```python
from build123d import *

# Parameters (mm, degrees)
F0_W     = 50.8
F0_H     = 76.2
F1_DEPTH = 12.7
F3_DEPTH = 6.35
F4_R     = 3.175
F5_DEPTH = 12.701


with BuildPart() as f1:
    # F0 (on Front) → F1 (new body)
    with BuildSketch(Plane.XZ):
        with Locations((25.4, 38.1)):
            Rectangle(F0_W, F0_H)
    extrude(amount=F1_DEPTH)

    # F2 (on face) → F3 (cut)
    with BuildSketch(Plane.XZ.offset(12.7)):
        with BuildLine():
            Line((22.225, 63.5), (0, 63.5))
            Line((0, 63.5), (0, 57.15))
            Line((0, 57.15), (15.896593, 57.15))
            ThreePointArc((15.896593, 57.15), (20.379061, 55.297775), (22.246556, 50.821648))
            Line((22.246556, 50.821648), (22.339729, 23.491532))
            Line((22.339729, 23.491532), (28.575, 23.61499))
            Line((28.575, 23.61499), (28.575, 57.15))
            ThreePointArc((28.575, 57.15), (26.715128, 61.640128), (22.225, 63.5))
        make_face()
    extrude(amount=-F3_DEPTH, mode=Mode.SUBTRACT)

    # F4 (on face) → F5 (cut, through all)
    with BuildSketch(Plane.XZ.offset(12.7)):
        with Locations((25.4, 69.85)):
            Circle(F4_R)
        with Locations((25.4, 6.35)):
            Circle(F4_R)
    extrude(amount=-F5_DEPTH, mode=Mode.SUBTRACT)


solid = f1.part
```
Geometry: final body of the model. Coordinates: model frame, mm. A direction names the side the tool comes from. Round coordinates to 2 decimals unless told otherwise and drop trailing zeros. Write each loop counter-clockwise with the first axis right and the second up, starting at its lowest first coordinate (ties: lowest second). Pieces come first, ordered by that corner, then holes. Notation, with made-up numbers: (46.25, 39) -> (89.25, 39) arc R32 cw to (89.25, 74) -> close; hole circle Ø1 at (-32.75, 62). An arc over 180 degrees is marked (long way). Return JSON: item names as keys, results as strings.
Q1. Set-up query: faces 4 (the flat face through (8, -10, 57.15)), 5 (the flat face through (31, -12.7, 39)), 6 (the flat face through (28.575, -10, 40)). Return all of +Z, -Z, +X, -X, +Y, -Y with unobstructed straight access to the full face (end or side cutting, diameter ignored); none if empty.
From the geometry:
{"face 4": "-X, -Y", "face 5": "+Z, -Z, +X, -X, -Y", "face 6": "-Y"}
Q2. Section A-A on z = 69.85. Return the cut outline in (x, y) (3 decimals), and give its area (3 significant figures).
From the geometry:
{"outline": "(0, -12.7) -> (22.225, -12.7) -> (22.225, 0) -> (0, 0) -> close; (28.575, -12.7) -> (50.8, -12.7) -> (50.8, 0) -> (28.575, 0) -> close", "area": "565 mm2"}
Q3. Section C-C on x = 8.5. Return the cut outline in (y, z), and give its area (3 significant figures).
From the geometry:
{"outline": "(-12.7, 0) -> (0, 0) -> (0, 76.2) -> (-12.7, 76.2) -> (-12.7, 63.5) -> (-6.35, 63.5) -> (-6.35, 57.15) -> (-12.7, 57.15) -> close", "area": "927 mm2"}
Q4. Section B-B on y = -8.5. Return the cut outline in (x, z) (3 decimals), and give its area (3 significant figures).
From the geometry:
{"outline": "(0, 0) -> (50.8, 0) -> (50.8, 76.2) -> (0, 76.2) -> (0, 63.5) -> (22.225, 63.5) arc R6.35 cw to (28.575, 57.15) -> (28.575, 23.615) -> (22.34, 23.492) -> (22.247, 50.822) arc R6.35 ccw to (15.897, 57.15) -> (0, 57.15) -> close; hole circle Ø6.35 at (25.4, 6.35); hole circle Ø6.35 at (25.4, 69.85)", "area": "3,410 mm2"}
Q5. Mould query, pull axis X, two halves, no side actions, for faces 1 (the flat face through (25, -6, 0)), 2 (the flat face through (23, -6.35, 50)), 3 (the cylindrical face through (26.764, -9.569, 61.59)). Classes: +X half, -X half, draft (parallel to the pull), parting line (faces both ways), or undercut.
From the geometry:
{"face 1": "draft", "face 2": "undercut", "face 3": "-X half"}
Q6. Section D-D on x = 25.4. Return the cut outline in (y, z) (3 decimals).
From the geometry:
{"outline": "(-12.7, 0) -> (0, 0) -> (0, 3.175) -> (-12.7, 3.175) -> close; (-12.7, 9.525) -> (0, 9.525) -> (0, 66.675) -> (-12.7, 66.675) -> (-12.7, 62.649) -> (-6.35, 62.649) -> (-6.35, 23.552) -> (-12.7, 23.552) -> close; (-12.7, 73.025) -> (0, 73.025) -> (0, 76.2) -> (-12.7, 76.2) -> close"}
Q7. Ray query, line 1 (Z direction, x = 25.4, y = -4.75) (3 decimals); line 2 (Z direction, x = 5.5, y = -11); line 3 (Z direction, x = 25.4, y = -7.75) (3 decimals). Return the intervals inside material, ascending.
From the geometry:
{"line 1": "0 to 3.175, 9.525 to 66.675, 73.025 to 76.2", "line 2": "0 to 57.15, 63.5 to 76.2", "line 3": "0 to 3.175, 9.525 to 23.552, 62.649 to 66.675, 73.025 to 76.2"}
